from build123d import *

# Parameters (mm, degrees)
F0_W     = 50.5
F0_H     = 16.5
F1_DEPTH = 5
F2_W     = 29.5
F2_H     = 8.8
F3_DEPTH = 23
F4_W     = 3
F4_H     = 1
F5_DEPTH = 28
F6_SIZE  = 0.5
F7_W     = 24.5
F7_H     = 5.5
F8_DEPTH = 23


with BuildPart() as f1:
    # F0 (on Front) → F1 (new body)
    with BuildSketch(Plane.XZ):
        with Locations((5.748162, 1.834772)):
            Rectangle(F0_W, F0_H)
    extrude(amount=F1_DEPTH)

    # F2 (on face) → F3 (join)
    with BuildSketch(Plane.XZ.offset(5)):
        with Locations((5.748162, 1.834772)):
            Rectangle(F2_W, F2_H)
    extrude(amount=F3_DEPTH)

    # F4 (on face) → F5 (cut)
    with BuildSketch(Plane.XZ.offset(28)):
        with Locations((-4.251838, 1.834772)):
            Rectangle(F4_W, F4_H)
        with Locations((0.748162, 1.834772)):
            Rectangle(F4_W, F4_H)
        with Locations((5.748162, 1.834772)):
            Rectangle(F4_W, F4_H)
        with Locations((10.748162, 1.834772)):
            Rectangle(F4_W, F4_H)
        with Locations((15.748162, 1.834772)):
            Rectangle(F4_W, F4_H)
    extrude(amount=-F5_DEPTH, mode=Mode.SUBTRACT)

    # F6
    f6_edges = [f1.edges().sort_by_distance(p)[0] for p in [
        (20.498162, -16.5, 6.234772),
        (-9.001838, -16.5, 6.234772),
        (20.498162, -16.5, -2.565228),
        (-9.001838, -16.5, -2.565228),
    ]]
    chamfer(f6_edges, length=F6_SIZE)

    # F7 (on face) → F8 (cut)
    with BuildSketch(Plane(origin=(0, 0, 0), x_dir=(-1, 0, 0), z_dir=(0, 1, 0))):
        with Locations((-5.748162, 1.834772)):
            Rectangle(F7_W, F7_H)
    extrude(amount=-F8_DEPTH, mode=Mode.SUBTRACT)


solid = f1.part
The model under review builds one solid part; all positions refer to its coordinate system, in mm. A direction names the side the tool comes from. Give positions to 0.01 mm unless a question says otherwise; leave off trailing zeros. Loops run counter-clockwise (first coordinate to the right, second up) from the corner with the lowest first, then second, coordinate; pieces in that order, holes last. Notation, with made-up numbers: (-29.5, -25) -> (2.5, -25) arc R30 ccw to (2.5, 10) -> close; hole circle Ø9 at (7, 14.5). An arc over 180 degrees is marked (long way). Put each result on its own line as item: value. Start each with the question number.
1. We need section B-B on x = -4.5. State the section outline as (y, z) points.
2. We need section D-D on x = 19. State the section outline as (y, z) points.
3. Wall thickness on probe 1 along X at (y, z) = (-22.5, -0.5); probe 2 along X at (y, z) = (-4.75, 4.5); probe 3 along Z at (x, y) = (8, -1.75): over which ranges is each line inside the solid? List them lowest first.
4. Clearance check with flat-ended pins moving along their axes: P1, Ø3, axis at y = -15, z = 4, coming from the -X side; P2, Ø1.5, axis at y = -6, z = 4.5, coming from the +X side; P3, Ø2.5, axis at x = 11, y = -25, coming from the +Z side. State where each tip first meets the part, or that it passes through.
5. Mouldability with a two-part tool opening along X and no side actions: class faces 4 (the face through (-9.002, -16, 2)), 5 (the face through (9.248, -26, 2)), 6 (the face through (5, -2, -6.415)) as released by +X, released by -X, zero draft, split by the parting line, or undercut.
6. We need section C-C on z = 3.5. State the section outline as (x, y) points.
7. For faces 1 (the face through (6, -16, 6.235)), 2 (the face through (6, -23, 1)), 3 (the face through (14.248, -26, 2)), list the 3-axis set-ups (+Z, -Z, +X, -X, +Y, -Y) from which the entire face can be reached by the end or side of a thin tool; tool diameter is ignored.
8. We need section A-A on y = -8. State the section outline as (x, z) points, then the cut area to 3 significant figures.
Determined:
1. outline: (-28, -2.57) -> (-5, -2.57) -> (-5, -6.42) -> (0, -6.42) -> (0, -0.92) -> (-23, -0.92) -> (-23, 1.33) -> (-28, 1.33) -> close; (-28, 2.33) -> (-23, 2.33) -> (-23, 4.58) -> (0, 4.58) -> (0, 10.08) -> (-5, 10.08) -> (-5, 6.23) -> (-28, 6.23) -> close
2. outline: (-28, -2.57) -> (-5, -2.57) -> (-5, -6.42) -> (0, -6.42) -> (0, 10.08) -> (-5, 10.08) -> (-5, 6.23) -> (-28, 6.23) -> close
3. probe 1: -9 to -6.5, 18 to 20.5
3. probe 2: -19.5 to -6.5, 18 to 31
3. probe 3: -6.42 to -0.92, 4.58 to 10.08
4. P1: x = -9
4. P2: x = 20.5
4. P3: z = 6.23
5. face 4: released by -X
5. face 5: undercut
5. face 6: zero draft
6. outline: (-19.5, -5) -> (-9, -5) -> (-9, -28) -> (20.5, -28) -> (20.5, -5) -> (31, -5) -> (31, 0) -> (18, 0) -> (18, -23) -> (-6.5, -23) -> (-6.5, 0) -> (-19.5, 0) -> close
7. face 1: +Z, +X, -X, -Y
7. face 2: +Y
7. face 3: +Y, -Y
8. outline: (-9, -2.07) -> (-8.5, -2.57) -> (20, -2.57) -> (20.5, -2.07) -> (20.5, 5.73) -> (20, 6.23) -> (-8.5, 6.23) -> (-9, 5.73) -> close; hole (-6.5, -0.92) -> (18, -0.92) -> (18, 4.58) -> (-6.5, 4.58) -> close
8. area: 124 mm^2
